from build123d import *

# Parameters (mm, degrees)
SKETCH_W  = 12.75
SKETCH_H  = 12.75
PAD_DEPTH = 10
FILLET_R  = 15


with BuildPart() as part:
    # Sketch → Pad (new body)
    with BuildSketch(Plane.XY):
        with BuildLine():
            ThreePointArc((25, 0), (0, 25), (-25, 0))
            Line((-25, 0), (-18.956776, -56.375))
            ThreePointArc((-18.956776, -56.375), (0, -70), (18.956776, -56.375))
            Line((18.956776, -56.375), (25, 0))
        make_face()
        Polygon((-17.525, 0), (-8.7625, -15.177095), (8.7625, -15.177095), (17.525, 0), (8.7625, 15.177095), (-8.7625, 15.177095), align=None, mode=Mode.SUBTRACT)
        with Locations((0, -50)):
            Rectangle(SKETCH_W, SKETCH_H, mode=Mode.SUBTRACT)
    extrude(amount=PAD_DEPTH)

    # Fillet
    fillet_edges = [part.edges().sort_by_distance(p)[0] for p in [
        (-25, 0, 5),
        (-18.956776, -56.375, 5),
        (18.956776, -56.375, 5),
        (25, 0, 5),
    ]]
    fillet(fillet_edges, radius=FILLET_R)


solid = part.part
The model under review builds one solid part; all positions refer to its coordinate system, in mm. A direction names the side the tool comes from. Coordinates: 2 decimals unless noted, no trailing zeros. Loops run counter-clockwise (first coordinate to the right, second up) from the corner with the lowest first, then second, coordinate; pieces in that order, holes last.
(1) Consider section B-B, the plane y = -3.5. Give the boundary of the cut face in (x, z), plus the area to 3 significant figures.
Determined:
outline: (-24.62, 0) - (-15.5, 0) - (-15.5, 10) - (-24.62, 10) - close; (15.5, 0) - (24.62, 0) - (24.62, 10) - (15.5, 10) - close
area: 182 mm2
(2) Insertion check: P1, Ø4, axis at x = -16, z = 8.5, coming from the -Y side; P2, Ø5, axis at x = 16.5, z = 4.5, coming from the +Y side; P3, Ø5, axis at y = -16, z = 2, coming from the -X side; P4, Ø3, axis at x = -9, y = -47.5, coming from the -Z side. Each pin has a flat end and moves straight along its axis. Give the tip position at first contact, or say it passes through.
Determined:
P1: stops at y = -64.28
P2: stops at y = 20.71
P3: stops at x = -23.55
P4: stops at z = 0
(3) Tool access review of faces 4 (the cylindrical face through (0.528, 24.994, 4.93)), 5 (the flat face through (-13.082, 7.695, 4.93)): name each direction out of +Z, -Z, +X, -X, +Y, -Y from which nothing blocks a thin tool from reaching the whole face with its end or side.
Determined:
face 4: +Z, -Z, +Y
face 5: +Z, -Z
(4) Wall thickness on L1, parallel to Y at x = 0, z = 8 (3 decimals); L2, parallel to Y at x = 1.5, z = 3.5 (3 decimals); L3, parallel to X at y = -48, z = 7 (3 decimals): over which ranges is each line inside the solid? List them lowest first.
Determined:
L1: y = -70 to -56.375, -43.625 to -15.177, 15.177 to 25
L2: y = -69.944 to -56.375, -43.625 to -15.177, 15.177 to 24.955
L3: x = -19.855 to -6.375, 6.375 to 19.855
(5) Draft analysis for pull direction X (two halves, no side actions). For faces 1 (the flat face through (6.375, -50, 5)), 2 (the cylindrical face through (18.5, -57.35, 5.07)), 3 (the cylindrical face through (-18.5, -57.35, 5.07)), state which applies: +X half, -X half, draft (parallel to the pull), parting line (faces both ways), or undercut.
Determined:
face 1: undercut
face 2: +X half
face 3: -X half
(6) Consider section D-D, the plane x = 12.5. Give the boundary of the cut face in (y, z).
Determined:
outline: (-65.61, 0) - (-8.7, 0) - (-8.7, 10) - (-65.61, 10) - close; (8.7, 0) - (21.65, 0) - (21.65, 10) - (8.7, 10) - close
(7) Consider section A-A, the plane x = 0. Give the boundary of the cut face in (y, z) (3 decimals), plus the area to 3 significant figures.
Determined:
outline: (-70, 0) - (-56.375, 0) - (-56.375, 10) - (-70, 10) - close; (-43.625, 0) - (-15.177, 0) - (-15.177, 10) - (-43.625, 10) - close; (15.177, 0) - (25, 0) - (25, 10) - (15.177, 10) - close
area: 519 mm2
